from build123d import *

# Parameters (mm, degrees)
CROQUIS1_R              = 1.5
CROQUIS1_R_2            = 2
CROQUIS1_R_3            = 5
CROQUIS1_R_4            = 3.5
SALIENTE_EXTRUIR1_DEPTH = 3


with BuildPart() as part:
    # Croquis1 → Saliente-Extruir1 (new body)
    with BuildSketch(Plane(origin=(0, 0, 0), x_dir=(1, 0, 0), z_dir=(0, 1, 0))):
        Polygon((0, 0), (15.75, 0), (15.75, 3), (23.75, 3), (31.75, 3), (31.75, 0), (47.5, 0), (47.5, 81), (31.75, 81), (31.75, 78), (23.75, 78), (15.75, 78), (15.75, 81), (0, 81), align=None)
        with Locations(Location((3.75, 49.25, 0), (0, 0, 270))):
            Circle(CROQUIS1_R, mode=Mode.SUBTRACT)
        with Locations(Location((3.75, 31.75, 0), (0, 0, 90))):
            Circle(CROQUIS1_R, mode=Mode.SUBTRACT)
        with Locations(Location((12.75, 40.5, 0), (0, 0, 270))):
            Circle(CROQUIS1_R_2, mode=Mode.SUBTRACT)
        with Locations(Location((23.75, 22, 0), (0, 0, 270))):
            Circle(CROQUIS1_R_3, mode=Mode.SUBTRACT)
        with Locations(Location((23.75, 40.5, 0), (0, 0, 270))):
            Circle(CROQUIS1_R_4, mode=Mode.SUBTRACT)
    extrude(amount=SALIENTE_EXTRUIR1_DEPTH)


solid = part.part
Work out the finished part from the listing and answer in its coordinate system (mm). A direction names the side the tool comes from. Round coordinates to 2 decimals unless told otherwise and drop trailing zeros. Loops run counter-clockwise (first coordinate to the right, second up) from the corner with the lowest first, then second, coordinate; pieces in that order, holes last. Notation, with made-up numbers: (64, 56) - (72, 56) arc R25 ccw to (72, 78) - close; hole circle Ø1 at (51, -16.5). An arc over 180 degrees is marked (long way). Use one line per item in the form item = value. Start each with the question number.
(1) Find section C-C on x = 12.75. Determine the outline of the cut face in (y, z).
(2) Find section D-D on y = 0.75. Determine the outline of the cut face in (x, z), and give its area (3 significant figures).
(3) Consider line 1 (X direction, y = 2.45, z = -40.5); line 2 (Z direction, x = 23.5, y = 0.9); line 3 (X direction, y = 2.3, z = -22). Determine where each line is inside the solid, lowest interval first.
(4) Find section B-B on z = -31.75. Determine the outline of the cut face in (x, y).
(5) Which of the six approach directions +Z, -Z, +X, -X, +Y, -Y give full straight-line access (tool end or side, diameter ignored) to faces 1 (the face through (14.102, 1.479, -41.974)), 2 (the face through (24, 1, -3)), 3 (the face through (31.75, 1, -80))?
(6) Flat-ended cylindrical pins translate along their axes: P1, Ø1.5, axis at x = 27.5, y = 1.5, coming from the +Z side; P2, Ø3, axis at x = 12.75, z = -40.5, coming from the -Y side; P3, Ø1.5, axis at x = 20, y = 2, coming from the -Z side. Find the tip coordinate at first contact, or state that the pin passes through.
(7) Find section A-A on x = 23.75. Determine the outline of the cut face in (y, z), and give its area (3 significant figures).
(8) Determine the mould class of faces 4 (the face through (23.904, 1.479, -43.997)), 5 (the face through (8, 1, -81)), 6 (the face through (47.5, 1, -40)) for opening direction X: +X half, -X half, draft (parallel to the pull), parting line (faces both ways), or undercut.
Answer list:
q1.outline = (0, -81) - (3, -81) - (3, -42.5) - (0, -42.5) - close; (0, -38.5) - (3, -38.5) - (3, 0) - (0, 0) - close
q2.outline = (0, -81) - (15.75, -81) - (15.75, -78) - (31.75, -78) - (31.75, -81) - (47.5, -81) - (47.5, 0) - (31.75, 0) - (31.75, -3) - (15.75, -3) - (15.75, 0) - (0, 0) - close; hole circle Ø3 at (3.75, -49.25); hole circle Ø3 at (3.75, -31.75); hole circle Ø4 at (12.75, -40.5); hole circle Ø10 at (23.75, -22); hole circle Ø7 at (23.75, -40.5)
q2.area = 3,610 mm^2
q3.line_1 = 0 to 10.75, 14.75 to 20.25, 27.25 to 47.5
q3.line_2 = -78 to -43.99, -37.01 to -26.99, -17.01 to -3
q3.line_3 = 0 to 18.75, 28.75 to 47.5
q4.outline = (0, 0) - (2.25, 0) - (2.25, 3) - (0, 3) - close; (5.25, 0) - (47.5, 0) - (47.5, 3) - (5.25, 3) - close
q5.face_1 = +Y, -Y
q5.face_2 = +Z, +Y, -Y
q5.face_3 = -Z, +Y, -Y
q6.P1 = -3
q6.P2 = through
q6.P3 = -78
q7.outline = (0, -78) - (3, -78) - (3, -44) - (0, -44) - close; (0, -37) - (3, -37) - (3, -27) - (0, -27) - close; (0, -17) - (3, -17) - (3, -3) - (0, -3) - close
q7.area = 174 mm^2
q8.face_4 = undercut
q8.face_5 = draft
q8.face_6 = +X half
